For this review, take the finished solid that the model builds, in its own axes (mm). Coordinates: 2 decimals unless noted, no trailing zeros. Order: outer loops, then holes, each group sorted by start corner. A loop starts at its lowest first (then second) coordinate and runs counter-clockwise, first axis right, second up. Notation, with made-up numbers: (-13, -20) -> (7, -20) arc R16 cw to (7, -16) -> close; hole circle Ø3 at (44, 61.25). An arc over 180 degrees is marked (long way). Answer as a JSON object with one key per item and string values. Group by question number.
1) Add section B-B, the plane x = -81. Write out the cut boundary in (y, z).
2) For pin 1 (4 mm diameter, centred on x = -67.5, y = 20, fed in from +Z); pin 2 (8 mm diameter, centred on x = -73, y = 9.5, fed in from +Z); pin 3 (3 mm diameter, centred on x = -75, y = 11.5, fed in from +Z), all flat-tipped, find the tip position at first contact; note any pin that passes through.
3) Add section A-A, the plane y = 18. Write out the cut boundary in (x, z).
4) Wall thickness on L1, parallel to Z at x = -51, y = 11; L2, parallel to Z at x = -71, y = 16.25: over which ranges is each line inside the solid? List them lowest first.
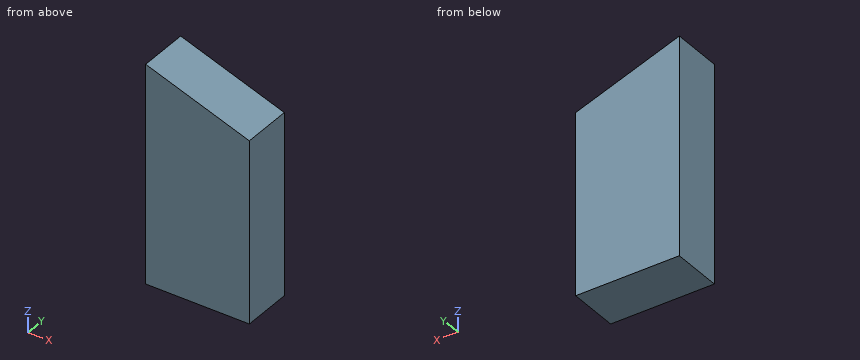
from build123d import *

# Parameters (mm, degrees)
F0_R     = 11
F1_DEPTH = 3.5
F3_DEPTH = 19.05


with BuildPart() as f1:
    # F0 (on Front) → F1 (new body, symmetric)
    with BuildSketch(Plane.XZ):
        with BuildLine():
            ThreePointArc((32.332994, 19.822553), (28.916134, 20.703546), (25.4, 21))
            Line((25.4, 21), (-85.4, 21))
            Line((-85.4, 21), (-85.4, -21))
            Line((-85.4, -21), (25.4, -21))
            ThreePointArc((25.4, -21), (46.103546, -3.516134), (32.332994, 19.822553))
        make_face()
        with Locations((-25.4, 0)):
            Circle(F0_R, mode=Mode.SUBTRACT)
        with Locations((25.4, 0)):
            Circle(F0_R, mode=Mode.SUBTRACT)
        with BuildLine():
            Line((-85.4, 21), (25.4, 21))
            ThreePointArc((25.4, 21), (28.916134, 20.703546), (32.332994, 19.822553))
            Line((32.332994, 19.822553), (-85.4, 61))
            Line((-85.4, 61), (-85.4, 21))
        make_face()
    extrude(amount=F1_DEPTH, both=True)


with BuildPart() as f3:
    # F2 (on face) → F3 (new body)
    with BuildSketch(Plane.XZ.offset(3.5)):
        Polygon((-46.4, 47.35964), (-85.4, 61), (-85.4, -21), (-46.4, -21), align=None)
    extrude(amount=F3_DEPTH)


with BuildPart() as f4_1:
    # F4: instance of F3
    add(f3.part.mirror(Plane.XZ))


solid = f4_1.part
Output values:
{
 "1": {"outline": "(3.5, -21) -> (22.55, -21) -> (22.55, 59.46) -> (3.5, 59.46) -> close"},
 "2": {"pin 1": "stops at z = 55.44", "pin 2": "stops at z = 58.06", "pin 3": "stops at z = 57.89"},
 "3": {"outline": "(-85.4, -21) -> (-46.4, -21) -> (-46.4, 47.36) -> (-85.4, 61) -> close"},
 "4": {"L1": "z = -21 to 48.97", "L2": "z = -21 to 55.96"}
}
